Input: part model. Units: mm. Frame: model coordinates. Give positions to 0.01 mm unless a question says otherwise; leave off trailing zeros. Loops run counter-clockwise (first coordinate to the right, second up) from the corner with the lowest first, then second, coordinate; pieces in that order, holes last. Notation, with made-up numbers: M 47.5,-18.75 L 54.5,-18.75 A28 ccw 54.5,9.25 Z; hole C 36.25,60.25 d4. An arc over 180 degrees is marked long. Use CSV: the item, a comma, the result in double quotes. Start each with the question number.
from build123d import *

# Parameters (mm, degrees)
SKETCH1_R           = 0.5
BOSS_EXTRUDE1_DEPTH = 1.57


with BuildPart() as part:
    # Sketch1 → Boss-Extrude1 (new body)
    with BuildSketch(Plane.XY):
        Polygon((13.7, 19.85), (-13.7, 19.85), (-13.7, -4.97), (-5, -27.8), (5, -27.8), (13.7, -4.97), align=None)
        with Locations((11.7, -2.43)):
            Circle(SKETCH1_R, mode=Mode.SUBTRACT)
        with Locations((11.7, 0.11)):
            Circle(SKETCH1_R, mode=Mode.SUBTRACT)
        with Locations((11.7, 2.65)):
            Circle(SKETCH1_R, mode=Mode.SUBTRACT)
        with Locations((11.7, 5.19)):
            Circle(SKETCH1_R, mode=Mode.SUBTRACT)
        with Locations((11.7, 7.73)):
            Circle(SKETCH1_R, mode=Mode.SUBTRACT)
        with Locations((11.7, 10.27)):
            Circle(SKETCH1_R, mode=Mode.SUBTRACT)
        with Locations((11.7, 12.81)):
            Circle(SKETCH1_R, mode=Mode.SUBTRACT)
        with Locations((11.7, 15.35)):
            Circle(SKETCH1_R, mode=Mode.SUBTRACT)
        with Locations((-11.7, 15.35)):
            Circle(SKETCH1_R, mode=Mode.SUBTRACT)
        with Locations((-11.7, -2.43)):
            Circle(SKETCH1_R, mode=Mode.SUBTRACT)
        with Locations((-11.7, 0.11)):
            Circle(SKETCH1_R, mode=Mode.SUBTRACT)
        with Locations((-11.7, 2.65)):
            Circle(SKETCH1_R, mode=Mode.SUBTRACT)
        with Locations((-11.7, 5.19)):
            Circle(SKETCH1_R, mode=Mode.SUBTRACT)
        with Locations((-11.7, 7.73)):
            Circle(SKETCH1_R, mode=Mode.SUBTRACT)
        with Locations((-11.7, 10.27)):
            Circle(SKETCH1_R, mode=Mode.SUBTRACT)
        with Locations((-11.7, 12.81)):
            Circle(SKETCH1_R, mode=Mode.SUBTRACT)
        with Locations((-1.27, -26.55)):
            Circle(SKETCH1_R, mode=Mode.SUBTRACT)
        with Locations((1.27, -26.55)):
            Circle(SKETCH1_R, mode=Mode.SUBTRACT)
    extrude(amount=BOSS_EXTRUDE1_DEPTH)


solid = part.part
Item 1: Mould query, pull axis X, two halves, no side actions, for faces 1 (the flat face through (-13.7, 8, 1)), 2 (the cylindrical face through (-12.2, -2.4, 0.8)), 3 (the flat face through (0, 19.85, 1)), 4 (the cylindrical face through (-12.2, 0.1, 0.8)). Classes: +X half, -X half, draft (parallel to the pull), parting line (faces both ways), or undercut.
Item 2: Section B-B (y = -2.43). Output: boundary loops of the cut face in (x, z).
Item 3: Section A-A (x = -1.27). Output: boundary loops of the cut face in (y, z).
Item 4: Section D-D (y = -26.55). Output: boundary loops of the cut face in (x, z).
Item 5: Section C-C (z = 1.3). State how many separate pieces and enclosed holes the cut face has, then the cut area to 3 significant figures.
Item 6: Material intervals for line 1 (X direction, y = 12.5, z = 0.85); line 2 (Y direction, x = 1.5, z = 0.3); line 3 (X direction, y = -23.5, z = 0.1), sorted ascending.
Recorded:
1,face 1,"-X half"
1,face 2,"undercut"
1,face 3,"draft"
1,face 4,"undercut"
2,outline,"M -13.7,0 L -12.2,0 L -12.2,1.57 L -13.7,1.57 Z; M -11.2,0 L 11.2,0 L 11.2,1.57 L -11.2,1.57 Z; M 12.2,0 L 13.7,0 L 13.7,1.57 L 12.2,1.57 Z"
3,outline,"M -27.8,0 L -27.05,0 L -27.05,1.57 L -27.8,1.57 Z; M -26.05,0 L 19.85,0 L 19.85,1.57 L -26.05,1.57 Z"
4,outline,"M -5.48,0 L -1.77,0 L -1.77,1.57 L -5.48,1.57 Z; M -0.77,0 L 0.77,0 L 0.77,1.57 L -0.77,1.57 Z; M 1.77,0 L 5.48,0 L 5.48,1.57 L 1.77,1.57 Z"
5,separate pieces,"1"
5,enclosed holes,"18"
5,area,"1,090 mm²"
6,line 1,"-13.7 to -12.09, -11.31 to 11.31, 12.09 to 13.7"
6,line 2,"-27.8 to -26.99, -26.11 to 19.85"
6,line 3,"-6.64 to 6.64"
